```python
from build123d import *

# Parameters (mm, degrees)
F1_DEPTH = 20
F2_W     = 10
F2_H     = 5
F3_DEPTH = 5.5
F4_W     = 10
F4_H     = 10
F5_DEPTH = 30.001
F6_W     = 5.5
F6_H     = 10
F7_DEPTH = 15.001


with BuildPart() as f1:
    # F0 (on Front) → F1 (new body)
    with BuildSketch(Plane.XZ):
        Polygon((0, 20), (0, 0), (30, 0), (30, 5), align=None)
    extrude(amount=F1_DEPTH)

    # F2 (on face) → F3 (cut)
    with BuildSketch(Plane.YZ.offset(30)):
        with Locations((-10, 2.5)):
            Rectangle(F2_W, F2_H)
    extrude(amount=-F3_DEPTH, mode=Mode.SUBTRACT)

    # F4 (on face) → F5 (cut, through all)
    with BuildSketch(Plane(origin=(0, 0, 0), x_dir=(0, -1, 0), z_dir=(-1, 0, 0))):
        with Locations((10, 15)):
            Rectangle(F4_W, F4_H)
    extrude(amount=-F5_DEPTH, mode=Mode.SUBTRACT)

    # F6 (on face) → F7 (cut, through all)
    with BuildSketch(Plane(origin=(0, 0, 5), x_dir=(1, 0, 0), z_dir=(0, 0, -1))):
        with Locations((27.25, 10)):
            Rectangle(F6_W, F6_H)
    extrude(amount=-F7_DEPTH, mode=Mode.SUBTRACT)


solid = f1.part
```
The listing builds one solid part. Answer for the finished solid, in the listing's coordinates (mm). A direction names the side the tool comes from. Coordinates: 2 decimals unless noted, no trailing zeros. Order: outer loops, then holes, each group sorted by start corner. A loop starts at its lowest first (then second) coordinate and runs counter-clockwise, first axis right, second up. Notation, with made-up numbers: M -15,48.25 L 9,48.25 A30 cw 9,71.25 Z; hole C 40.25,-29.5 d4. An arc over 180 degrees is marked long. Answer as a JSON object with one key per item and string values. Group by question number.
1. Section A-A on z = 12.75 is taken. Write down the section's boundary in (x, y).
2. Section B-B on x = 12 is taken. Write down the section's boundary in (y, z).
3. Flat-ended cylindrical pins translate along their axes: P1, Ø4, axis at y = -8, z = 9.5, coming from the +X side; P2, Ø3, axis at x = 5.5, y = -10.5, coming from the +Z side; P3, Ø10, axis at x = 17.5, y = -2.5, coming from the +Z side. Find the tip coordinate at first contact, or state that the pin passes through.
4. A tool of negligible diameter and unlimited length cuts with its end or side. For faces 1 (the flat face through (15, -10, 0)), 2 (the flat face through (24.5, -10, 4)), 3 (the flat face through (8, -5, 14)), from which of +Z, -Z, +X, -X, +Y, -Y can it reach the whole face along a straight path? Write none if from no direction.
5. Section D-D on y = -12 is taken. Write down the section's boundary in (x, z), then the cut area to 3 significant figures.
6. Section C-C on z = 18.25 is taken. Write down the section's boundary in (x, y), then the cut area to 3 significant figures.
7. Determine the mould class of faces 4 (the flat face through (11, 0, 8)), 5 (the flat face through (30, -2, 2)), 6 (the flat face through (27, -15, 3)), 7 (the flat face through (10, -10, 10)) for opening direction Y: released by +Y, released by -Y, zero draft, split by the parting line, or undercut.
8. Straight lines are drawn through the part: line 1 (Y direction, x = 28, z = 1.5); line 2 (X direction, y = -14, z = 7.25); line 3 (Z direction, x = 10, y = -13.25). For each, find the intervals that lie inside material, in ascending order.
Values follow:
{
 "1": {"outline": "M 0,-20 L 14.5,-20 L 14.5,-15 L 0,-15 Z; M 0,-5 L 14.5,-5 L 14.5,0 L 0,0 Z"},
 "2": {"outline": "M -20,0 L 0,0 L 0,14 L -5,14 L -5,10 L -15,10 L -15,14 L -20,14 Z"},
 "3": {"P1": "x = 24.5", "P2": "z = 10", "P3": "z = 13.75"},
 "4": {"face 1": "-Z, +X, -X, +Y, -Y", "face 2": "+Z, -Z, +X", "face 3": "+Z, +X, -X"},
 "5": {"outline": "M 0,0 L 24.5,0 L 24.5,7.75 L 20,10 L 0,10 Z", "area": "240 mm2"},
 "6": {"outline": "M 0,-20 L 3.5,-20 L 3.5,-15 L 0,-15 Z; M 0,-5 L 3.5,-5 L 3.5,0 L 0,0 Z", "area": "35.0 mm2"},
 "7": {"face 4": "released by +Y", "face 5": "zero draft", "face 6": "undercut", "face 7": "undercut"},
 "8": {"line 1": "-20 to -15, -5 to 0", "line 2": "0 to 24.5", "line 3": "0 to 10"}
}
